The listing builds one solid part. Answer for the finished solid, in the listing's coordinates (mm). A direction names the side the tool comes from. Give positions to 0.01 mm unless a question says otherwise; leave off trailing zeros. Write each loop counter-clockwise with the first axis right and the second up, starting at its lowest first coordinate (ties: lowest second). Pieces come first, ordered by that corner, then holes. Notation, with made-up numbers: (-2.5, -25) -> (19.5, -25) arc R20 ccw to (19.5, 8) -> close; hole circle Ø11 at (4, 44). An arc over 180 degrees is marked (long way). Use CSV: the item, a comma, the result in double quotes. Start each with the question number.
from build123d import *

# Parameters (mm, degrees)
SKETCH1_R           = 2
BOSS_EXTRUDE1_DEPTH = 12
CUT_EXTRUDE1_DEPTH  = 162.777588211
SKETCH5_R           = 2
BOSS_EXTRUDE3_DEPTH = 4
CUT_EXTRUDE2_DEPTH  = 12.5
CHAMFER1_SIZE       = 3
FILLET1_R           = 4
CUT_EXTRUDE3_DEPTH  = 156.224708777
CUT_EXTRUDE4_DEPTH  = 156.224708777


with BuildPart() as part:
    # Sketch1 → Boss-Extrude1 (new, symmetric)
    with BuildSketch(Plane(origin=(0, 0, 0), x_dir=(0, 0, -1), z_dir=(1, 0, 0))):
        with BuildLine():
            Line((-121.907859823, 4), (-145.256630116, -4.68622038))
            ThreePointArc((-145.256630116, -4.68622038), (-151.290045259, -2.568172828), (-150.306967189, 3.75019573))
            Line((-150.306967189, 3.75019573), (-133.491442782, 18.578325107))
            Line((-133.491442782, 18.578325107), (-0.653491001, 30.01252535))
            Line((-0.653491001, 30.01252535), (41.089036304, 23.188119662))
            Line((41.089036304, 23.188119662), (61.107888441, 4.370001963))
            ThreePointArc((61.107888441, 4.370001963), (61.822541623, -3.565775777), (54.025769542, -5.208225973))
            Line((54.025769542, -5.208225973), (42.456256278, 1.398706774))
            ThreePointArc((42.456256278, 1.398706774), (37.66895292, 3.361815488), (32.53825078, 4.031117219))
            Line((32.53825078, 4.031117219), (16.022685374, 4.031117219))
            ThreePointArc((16.022685374, 4.031117219), (14.241499513, 3.602468352), (12.850348738, 2.410385115))
            Line((12.850348738, 2.410385115), (7.292636005, -5.274226019))
            ThreePointArc((7.292636005, -5.274226019), (2.262889815, -8.71087422), (-3.803564356, -8.156770083))
            Line((-3.803564356, -8.156770083), (-25.855369948, 2.126155741))
            ThreePointArc((-25.855369948, 2.126155741), (-29.978942905, 3.525920142), (-34.307735183, 4))
            Line((-34.307735183, 4), (-121.907859823, 4))
        make_face()
        Circle(SKETCH1_R, mode=Mode.SUBTRACT)
        with Locations((57, 0)):
            Circle(SKETCH1_R, mode=Mode.SUBTRACT)
        with Locations((-147, 0)):
            Circle(SKETCH1_R, mode=Mode.SUBTRACT)
    extrude(amount=BOSS_EXTRUDE1_DEPTH, both=True)

    # Sketch2 → Cut-Extrude1 (cut, through all)
    with BuildSketch(Plane(origin=(0, 29.127166191, -4.761944507), x_dir=(1, 0, 0), z_dir=(0, 0.9868978946219392, -0.16134604299698216))):
        Polygon((3.5, 62.250818245), (3.5, 52.064388241), (-12, 17.250818245), (-12, 62.250818245), align=None)
    extrude(amount=-CUT_EXTRUDE1_DEPTH, mode=Mode.SUBTRACT)

    # Sketch5 → Boss-Extrude3 (add)
    with BuildSketch(Plane.ZY.offset(12)):
        with BuildLine():
            Line((145.256630116, -4.68622038), (121.907859823, 4))
            Line((121.907859823, 4), (108.907859823, 4))
            Line((108.907859823, 4), (120.491442782, 19.697317091))
            Line((120.491442782, 19.697317091), (133.491442782, 18.578325107))
            Line((133.491442782, 18.578325107), (150.306967189, 3.75019573))
            ThreePointArc((150.306967189, 3.75019573), (151.290045259, -2.568172828), (145.256630116, -4.68622038))
        make_face()
        with Locations((147, 0)):
            Circle(SKETCH5_R, mode=Mode.SUBTRACT)
    extrude(amount=BOSS_EXTRUDE3_DEPTH)

    # Sketch6 → Cut-Extrude2 (cut)
    with BuildSketch(Plane(origin=(4, 0, 0), x_dir=(0, 0, -1), z_dir=(1, 0, 0))):
        with BuildLine():
            Line((-150.306967189, 3.75019573), (-138.821377712, 13.878325107))
            Line((-138.821377712, 13.878325107), (50.992864285, 13.878325107))
            Line((50.992864285, 13.878325107), (61.107888441, 4.370001963))
            ThreePointArc((61.107888441, 4.370001963), (61.822541623, -3.565775777), (54.025769542, -5.208225973))
            Line((54.025769542, -5.208225973), (42.456256278, 1.398706774))
            ThreePointArc((42.456256278, 1.398706774), (37.66895292, 3.361815488), (32.53825078, 4.031117219))
            Line((32.53825078, 4.031117219), (16.022685374, 4.031117219))
            ThreePointArc((16.022685374, 4.031117219), (14.241499513, 3.602468352), (12.850348738, 2.410385115))
            Line((12.850348738, 2.410385115), (7.292636005, -5.274226019))
            ThreePointArc((7.292636005, -5.274226019), (2.262889815, -8.71087422), (-3.803564356, -8.156770083))
            Line((-3.803564356, -8.156770083), (-25.855369948, 2.126155741))
            ThreePointArc((-25.855369948, 2.126155741), (-29.978942905, 3.525920142), (-34.307735183, 4))
            Line((-34.307735183, 4), (-121.907859823, 4))
            Line((-121.907859823, 4), (-145.256630116, -4.68622038))
            ThreePointArc((-145.256630116, -4.68622038), (-151.290045259, -2.568172828), (-150.306967189, 3.75019573))
        make_face()
    extrude(amount=-CUT_EXTRUDE2_DEPTH, mode=Mode.SUBTRACT)

    # Chamfer1
    chamfer1_edges = [part.edges().sort_by_distance(p)[0] for p in [
        (-16, 11.848658545, 114.699651303),
    ]]
    chamfer(chamfer1_edges, length=CHAMFER1_SIZE)

    # Fillet1
    # the kernel refuses this fillet: 4 mm, written as the material it adds along each edge
    with BuildSketch(Plane(origin=(-12, -1.322167469, 104.980451844), x_dir=(-1, 0, 0), z_dir=(0, 0.8046360890172893, 0.593768274877465))) as fillet1_piece_1_section:
        with BuildLine():
            CenterArc((4, -2.645751311), FILLET1_R, 138.590377891, 41.409622109)
            Line((0, -2.645751311), (0, 0))
            Line((0, 0), (1, 0))
        make_face()
    fillet1_piece_1 = extrude(amount=32.737348458, mode=Mode.PRIVATE)
    fillet1_piece_1 = split(fillet1_piece_1, bisect_by=Plane(origin=(-12, 20.868035787, 106.890502579), z_dir=(0, -0.9963158941582452, -0.08575919220501364)), keep=Keep.TOP, mode=Mode.PRIVATE)
    fillet1_piece_1 = split(fillet1_piece_1, bisect_by=Plane(origin=(-12, 4, 104.980451844), z_dir=(0, 1, 0)), keep=Keep.TOP, mode=Mode.PRIVATE)
    add(fillet1_piece_1)
    # the kernel refuses this fillet: 4 mm, written as the material it takes off along each edge
    with BuildSketch(Plane(origin=(-16, 0.667088192, 110.176784644), x_dir=(0, -0.593768274877465, 0.8046360890172894), z_dir=(0, 0.8046360890172893, 0.593768274877465))) as fillet1_2_piece_1:
        with BuildLine():
            CenterArc((FILLET1_R * 0.414213562373, FILLET1_R), FILLET1_R, 225, 45)
            Line((-FILLET1_R * 0.292893218813, FILLET1_R * 0.292893218813), (0, 0))
            Line((0, 0), (FILLET1_R * 0.414213562373, 0))
        make_face()
    extrude(amount=27.417837682, mode=Mode.SUBTRACT)

    # Sketch7 → Cut-Extrude3 (cut, through all)
    with BuildSketch(Plane(origin=(0, 29.847630452, 2.569173785), x_dir=(1, 0, 0), z_dir=(0, 0.9963158941582453, 0.08575919220501363))):
        Polygon((12, -111.406384024), (8, -100.416474347), (8, -40.655449605), (12, -20.077233541), align=None)
    extrude(amount=-CUT_EXTRUDE3_DEPTH, mode=Mode.SUBTRACT)

    # Sketch8 → Cut-Extrude4 (cut, through all)
    with BuildSketch(Plane(origin=(0, 29.847630452, 2.569173785), x_dir=(1, 0, 0), z_dir=(0, 0.9963158941582453, 0.08575919220501363))):
        with BuildLine():
            Line((-5.5, -42.241808783), (-5.5, -23.077233541))
            ThreePointArc((-5.5, -23.077233541), (-2, -19.577233541), (1.5, -23.077233541))
            Line((1.5, -23.077233541), (1.5, -42.241808783))
            ThreePointArc((1.5, -42.241808783), (-2, -45.741808783), (-5.5, -42.241808783))
        make_face()
        with BuildLine():
            Line((-5.5, -86.406384024), (-5.5, -67.241808783))
            ThreePointArc((-5.5, -67.241808783), (-2, -63.741808783), (1.5, -67.241808783))
            Line((1.5, -67.241808783), (1.5, -86.406384024))
            ThreePointArc((1.5, -86.406384024), (-2, -89.906384024), (-5.5, -86.406384024))
        make_face()
    extrude(amount=-CUT_EXTRUDE4_DEPTH, mode=Mode.SUBTRACT)


solid = part.part
Q1. Section C-C on z = 31 is taken. Give the vertices of the cut face in (x, y), then the cut area to 3 significant figures.
Q2. For faces 1 (the face through (-11, 4, 77)), 2 (the face through (1.5, 18, 79)), 3 (the face through (-12.266, 11.662, 113.055)), 4 (the face through (-1.923, 19.838, 47.618)), 5 (the face through (2, 13.878, 45)), determine the directions among +Z, -Z, +X, -X, +Y, -Y from which every point of the face is accessible in a straight line to the end or side of a thin tool.
Q3. The mould has two halves that part along Z. Classify faces 6 (the face through (8, 0, 149)), 7 (the face through (-12, 15, 31)), 8 (the face through (8, 4.031, -24)), 9 (the face through (-13.9, 11.65, 115.67)): +Z half, -Z half, draft (parallel to the pull), parting line (faces both ways), or undercut.
Q4. Flat-ended cylindrical pins translate along their axes: pin 1 Ø18.5 at (y, z) = (7.5, 85) entering from +X; pin 2 Ø3 at (x, z) = (-9.5, -22.5) entering from -Y; pin 3 Ø4 at (y, z) = (21, -5.5) entering from -X. Find the tip coordinate at first contact, or state that the pin passes through.
Q5. Section A-A on z = -57 is taken. Give the vertices of the cut face in (x, y), then the cut area to 3 significant figures.
Q6. Section B-B on z = 57 is taken. Give the vertices of the cut face in (x, y).
Q7. Straight lines are drawn through the part: L1, parallel to X at y = 7, z = 41.5; L2, parallel to Z at x = -3.5, y = 15; L3, parallel to X at y = 6.5, z = -4. For each, find the intervals that lie inside material, in ascending order.
Output:
1,outline,"(-12, 3.72) -> (-8.5, 3.72) -> (-8.5, 13.88) -> (-5.5, 13.88) -> (-5.5, 27.4) -> (-12, 27.4) -> close; (1.5, 13.88) -> (4, 13.88) -> (4, 3.72) -> (9.96, 3.72) -> (10.36, 27.4) -> (1.5, 27.4) -> close"
1,area,"303 mm²"
2,face 1,"+X, -X, -Y"
2,face 2,"+Y, -Y"
2,face 3,"-Z, -X, +Y"
2,face 4,"+Y"
2,face 5,"+Z, -Z, -Y"
3,face 6,"undercut"
3,face 7,"draft"
3,face 8,"undercut"
3,face 9,"-Z half"
4,pin 1,"x = 8"
4,pin 2,"y = 4.03"
4,pin 3,"x = -12"
5,outline,"(4, -6) -> (12, -6) -> (12, -2) -> (4, -2) -> close; (4, 2) -> (12, 2) -> (12, 8.23) -> (4, 8.23) -> close"
5,area,"81.8 mm²"
6,outline,"(-12, 4) -> (-8.5, 4) -> (-8.5, 13.88) -> (4, 13.88) -> (4, 4) -> (8, 4) -> (8, 25.16) -> (-12, 25.16) -> close"
7,L1,"-12 to -8.5, 4 to 8"
7,L2,"-39.28 to 21.28, 46.86 to 65.61, 91.19 to 137.55"
7,L3,"-12 to -8.5, 4 to 12"
